Can you work these out from the model? Positions are in its coordinate system, mm. A direction names the side the tool comes from. Round coordinates to 2 decimals unless told otherwise and drop trailing zeros. Write each loop counter-clockwise with the first axis right and the second up, starting at its lowest first coordinate (ties: lowest second). Pieces come first, ordered by that corner, then holes. Notation, with made-up numbers: M 65,-6 L 89,-6 A21 cw 89,9 Z; hole C 64,85 d3. An arc over 180 degrees is marked long. Answer in a Markdown table with one row per item. Add a question column.
(1) If I drill on probe 1 along Z at (x, y) = (0, 1.1); probe 2 along Z at (x, y) = (0, 0.7); probe 3 along X at (y, z) = (0.8, 0), over which ranges is the centre line in solid material (lowest first)?
(2) Suppose I cut it at B-B, the plane x = 0. Write out the boundary of the cut face in (y, z).
(3) For faces 1 (the face through (-1.2, 0, 1.2)), 2 (the face through (-0.54, 1.49, 2.44)), which set-ups out of +Z, -Z, +X, -X, +Y, -Y let a thin tool reach every point of the face, with its end or its side?
(4) Suppose I cut it at A-A, the plane z = 0. Write out the boundary of the cut face in (x, y).
(5) Suppose I cut it at D-D, the plane y = 1.45. Write out the boundary of the cut face in (x, z).
(6) Suppose I cut it at C-C, the plane y = 0.5. Write out the boundary of the cut face in (x, z), then the cut area to 3 significant figures.
(7) I'm going to push a flat-ended pin straight in: pin 1 (2 mm diameter, centred on x = -4, z = -3, fed in from +Y). Where does the tip first touch, or does it pass through?
from build123d import *

# Parameters (mm, degrees)
PAD001_DEPTH    = 1
SKETCH004_R     = 2.5
PAD002_DEPTH    = 1
SKETCH005_R     = 1.5
POCKET002_DEPTH = 2.001


with BuildPart() as part:
    # Sketch003 → Pad001 (new body)
    with BuildSketch(Plane.XZ):
        with BuildLine():
            Line((-3.5, 5), (3.5, 5))
            ThreePointArc((6, 1), (5.323593, 3.358495), (3.5, 5))
            Line((6, 1), (6, -1))
            ThreePointArc((3.5, -5), (5.323593, -3.358495), (6, -1))
            Line((3.5, -5), (-3.5, -5))
            ThreePointArc((-6, -1), (-5.323593, -3.358495), (-3.5, -5))
            Line((-6, -1), (-6, 1))
            ThreePointArc((-3.5, 5), (-5.323593, 3.358495), (-6, 1))
        make_face()
    extrude(amount=-PAD001_DEPTH)

    # Sketch004 (on Face10 of Pad001) → Pad002 (join)
    with BuildSketch(Plane(origin=(0, 1, 0), x_dir=(1, 0, 0), z_dir=(0, 1, 0))):
        Circle(SKETCH004_R)
    extrude(amount=PAD002_DEPTH)

    # Sketch005 (on Face12 of Pad002) → Pocket002 (cut, through all)
    with BuildSketch(Plane(origin=(0, 2, 0), x_dir=(1, 0, 0), z_dir=(0, 1, 0))):
        Circle(SKETCH005_R)
    extrude(amount=-POCKET002_DEPTH, mode=Mode.SUBTRACT)


solid = part.part
Calculated:
| question | item | result |
|---|---|---|
| 1 | probe 1 | -2.5 to -1.5, 1.5 to 2.5 |
| 1 | probe 2 | -5 to -1.5, 1.5 to 5 |
| 1 | probe 3 | -6 to -1.5, 1.5 to 6 |
| 2 | outline | M 0,-5 L 1,-5 L 1,-2.5 L 2,-2.5 L 2,-1.5 L 0,-1.5 Z; M 0,1.5 L 2,1.5 L 2,2.5 L 1,2.5 L 1,5 L 0,5 Z |
| 3 | face 1 | +Z, -Z, +X, -X, -Y |
| 3 | face 2 | +Y |
| 4 | outline | M -6,0 L -1.5,0 L -1.5,2 L -2.5,2 L -2.5,1 L -6,1 Z; M 1.5,0 L 6,0 L 6,1 L 2.5,1 L 2.5,2 L 1.5,2 Z |
| 5 | outline | C 0,0 d5; hole C 0,0 d3 |
| 6 | outline | M -6,-1 A4.45 ccw -3.5,-5 L 3.5,-5 A4.45 ccw 6,-1 L 6,1 A4.45 ccw 3.5,5 L -3.5,5 A4.45 ccw -6,1 Z; hole C 0,0 d3 |
| 6 | area | 102 mm² |
| 7 | pin 1 | y = 1 |
